Part model, mm, in its own coordinate system. Face numbers are marked on the shaded views. A direction names the side the tool comes from. Round coordinates to 2 decimals unless told otherwise and drop trailing zeros. Write each loop counter-clockwise with the first axis right and the second up, starting at its lowest first coordinate (ties: lowest second). Pieces come first, ordered by that corner, then holes. Notation, with made-up numbers: M -38.5,8.5 L -0.5,8.5 A28 ccw -0.5,47.5 Z; hole C 89,55 d10. An arc over 180 degrees is marked long. Use one line per item in the form item = value. Start each with the question number.
Item 1: Mould opens along X. For the marked faces 4, 5 and 6 say: +X half, -X half, draft (parallel to the pull), parting line (faces both ways), or undercut.
Item 2: Flat gauge pins, fed straight in: pin 1 Ø6 at (x, z) = (1.5, -4.5) entering from -Y; pin 2 Ø8 at (y, z) = (-7, 3.5) entering from -X; pin 3 Ø8 at (x, z) = (-10.5, 0) entering from +Y. Where does each tip first touch, or does it go through?
Item 3: Cut at B-B, the plane z = 5.75. Give the cut face in (x, y), then the cut area to 3 significant figures.
Item 4: Probe L1, parallel to X at y = 0.3, z = -6; L2, parallel to Y at x = -0.25, z = -6.5; L3, parallel to X at y = -9, z = -1. List the from-to ranges inside material, lowest first.
Item 5: Cut at A-A, the plane x = 12.15. Give the cut face in (y, z), then the cut area to 3 significant figures.
Item 6: Cut at D-D, the plane y = 3. Give the cut face in (x, z).
Item 7: Cut at C-C, the plane z = 2. Give the cut face in (x, y).
Item 8: Which spindle directions (+Z, -Z, +X, -X, +Y, -Y) get a long thin tool onto all of the face, cutting with end or side? Do the marked faces 1, 2 and 3. Say none if no direction does.
from build123d import *

# Parameters (mm, degrees)
SKETCH_1_W          = 29.3
SKETCH_1_H          = 17
EXTRUDE_1_DEPTH     = 1.5
SKETCH_2_R          = 1.25
CUT_EXTRUDE_1_DEPTH = 18.003602559
SKETCH_4_W          = 6.098514982
SKETCH_4_H          = 2.670072728
EXTRUDE_2_DEPTH     = 4
SKETCH_5_R          = 4.492338227
SKETCH_5_R_2        = 4.429267197
EXTRUDE_3_DEPTH     = 10
SKETCH_6_R          = 2.746946082
EXTRUDE_4_DEPTH     = 2
FILLET_1_R          = 1


with BuildPart() as part:
    # 草图1 → 凸台-拉伸1 (new body)
    with BuildSketch(Plane(origin=(0, 0, 0), x_dir=(1, 0, 0), z_dir=(0, 1, 0))):
        Rectangle(SKETCH_1_W, SKETCH_1_H)
    extrude(amount=EXTRUDE_1_DEPTH)

    # 草图2 → 切除-拉伸1 (cut, through all)
    with BuildSketch(Plane(origin=(0, 1.5, 0), x_dir=(1, 0, 0), z_dir=(0, 1, 0))):
        with Locations(Location((-12.15, 6, 0), (0, 0, 270))):
            Circle(SKETCH_2_R)
        with Locations(Location((12.15, 6, 0), (0, 0, 90))):
            Circle(SKETCH_2_R)
        with Locations(Location((12.15, -6, 0), (0, 0, 270))):
            Circle(SKETCH_2_R)
        with Locations(Location((-12.15, -6, 0), (0, 0, 90))):
            Circle(SKETCH_2_R)
    extrude(amount=-CUT_EXTRUDE_1_DEPTH, mode=Mode.SUBTRACT)

    # 草图4 → 凸台-拉伸2 (add)
    with BuildSketch(Plane.XY.offset(8.5)):
        with Locations((-3.14217972, 2.835036364)):
            Rectangle(SKETCH_4_W, SKETCH_4_H)
    extrude(amount=-EXTRUDE_2_DEPTH)

    # 草图5 → 凸台-拉伸3 (add)
    with BuildSketch(Plane.XZ):
        with Locations(Location((-4.961846609, 2.903857851, 0), (0, 0, 90))):
            Circle(SKETCH_5_R)
        with Locations(Location((5.295992796, 2.903857851, 0), (0, 0, 90))):
            Circle(SKETCH_5_R_2)
    extrude(amount=EXTRUDE_3_DEPTH)

    # 草图6 → 凸台-拉伸4 (add)
    with BuildSketch(Plane.XZ):
        with Locations(Location((0, -5.440327707, 0), (0, 0, 90))):
            Circle(SKETCH_6_R)
    extrude(amount=EXTRUDE_4_DEPTH)

    # 圆角1
    fillet_1_edges = [part.edges().sort_by_distance(p)[0] for p in [
        (14.65, 0.75, 8.5),
        (-14.65, 0.75, 8.5),
        (-14.65, 0.75, -8.5),
        (14.65, 0.75, -8.5),
    ]]
    fillet(fillet_1_edges, radius=FILLET_1_R)


solid = part.part
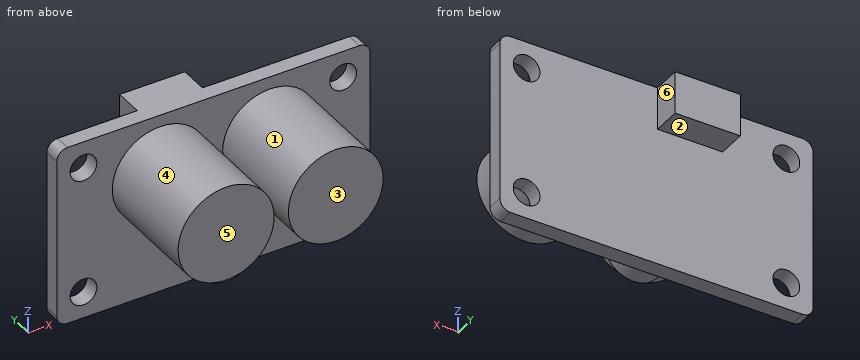
Model answer:
q1.face_4 = undercut
q1.face_5 = draft
q1.face_6 = +X half
q2.pin_1 = -2
q2.pin_2 = -9.45
q2.pin_3 = 1.5
q3.outline = M -14.65,0 L -13.37,0 L -13.37,1.5 L -14.65,1.5 Z; M -10.93,0 L -8.44,0 L -8.44,-10 L -1.49,-10 L -1.49,0 L 1.9,0 L 1.9,-10 L 8.69,-10 L 8.69,0 L 10.93,0 L 10.93,1.5 L -0.09,1.5 L -0.09,4.17 L -6.19,4.17 L -6.19,1.5 L -10.93,1.5 Z; M 13.37,0 L 14.65,0 L 14.65,1.5 L 13.37,1.5 Z
q3.area = 190 mm²
q4.L1 = -14.65 to -13.4, -10.9 to 10.9, 13.4 to 14.65
q4.L2 = -2 to 1.5
q4.L3 = -7.18 to -2.74, 3.2 to 7.39
q5.outline = M 0,-8.5 L 1.5,-8.5 L 1.5,-7.25 L 0,-7.25 Z; M 0,-4.75 L 1.5,-4.75 L 1.5,4.75 L 0,4.75 Z; M 0,7.25 L 1.5,7.25 L 1.5,8.5 L 0,8.5 Z
q5.area = 18.0 mm²
q6.outline = M -6.19,4.5 L -0.09,4.5 L -0.09,8.5 L -6.19,8.5 Z
q7.outline = M -14.65,0 L -9.36,0 L -9.36,-10 L -0.56,-10 L -0.56,0 L 0.96,0 L 0.96,-10 L 9.63,-10 L 9.63,0 L 14.65,0 L 14.65,1.5 L -14.65,1.5 Z
q8.face_1 = -Y
q8.face_2 = -Z, +X, -X, +Y
q8.face_3 = +Z, -Z, +X, -X, -Y
